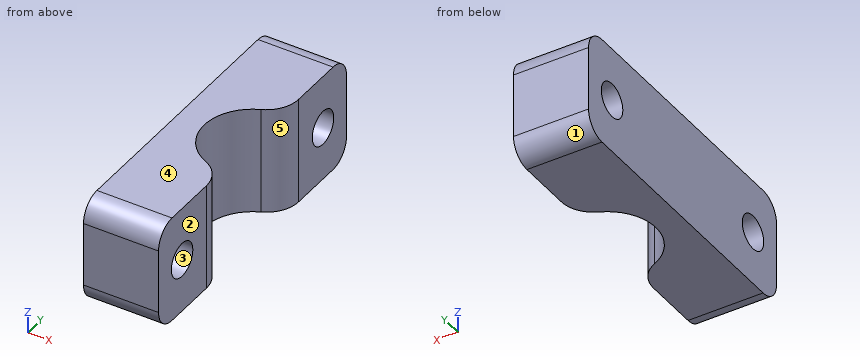
from build123d import *

# Parameters (mm, degrees)
SKETCH1_W               = 12
SKETCH1_H               = 2.1
BOSS_EXTRUDE1_DEPTH     = 3
BOSS_EXTRUDE1_2_DEPTH   = 3
SKETCH2_W               = 4
SKETCH2_H               = 6
BOSS_EXTRUDE2_DEPTH     = 6
SKETCH3_W               = 7
SKETCH3_H               = 28
BOSS_EXTRUDE3_DEPTH     = 5
CUT_EXTRUDE1_DEPTH      = 25.108425983
CUT_EXTRUDE1_DEPTH_BACK = 25.108425983
SKETCH5_R               = 4.5
FILLET1_R               = 3
FILLET2_R               = 2
SKETCH6_R               = 1.6
CUT_EXTRUDE2_DEPTH      = 16
SKETCH7_W               = 18.107499601
SKETCH7_H               = 21.771661969
CUT_EXTRUDE3_DEPTH      = 30


with BuildPart() as part:
    # Sketch1 → Boss-Extrude1 (new, symmetric)
    with BuildSketch(Plane.XY):
        with Locations((0, 1.95)):
            Rectangle(SKETCH1_W, SKETCH1_H)
    extrude(amount=BOSS_EXTRUDE1_DEPTH, both=True)


with BuildPart() as body_2:
    # Sketch1 → Boss-Extrude1 2 (new, symmetric)
    with BuildSketch(Plane.XY):
        with Locations((0, -1.95)):
            Rectangle(SKETCH1_W, SKETCH1_H)
    extrude(amount=BOSS_EXTRUDE1_2_DEPTH, both=True)


with BuildPart() as body_3:
    # Sketch2 → Boss-Extrude2 (new body)
    with BuildSketch(Plane.XY.offset(3)):
        with Locations((8, 0)):
            Rectangle(SKETCH2_W, SKETCH2_H)
    extrude(amount=-BOSS_EXTRUDE2_DEPTH)

    # Sketch3 → Boss-Extrude3 (add, symmetric)
    with BuildSketch(Plane.XY):
        with Locations((13.388345193, 0)):
            Rectangle(SKETCH3_W, SKETCH3_H)
    extrude(amount=BOSS_EXTRUDE3_DEPTH, both=True)

    # Sketch5 → Cut-Extrude1 (cut, two sides: drawn at the far end of the back side and taken through both)
    with BuildSketch(Plane.XY.offset(5).offset(-CUT_EXTRUDE1_DEPTH_BACK)):
        with Locations((16.888345193, 0)):
            Circle(SKETCH5_R)
    extrude(amount=CUT_EXTRUDE1_DEPTH + CUT_EXTRUDE1_DEPTH_BACK, mode=Mode.SUBTRACT)

    # Fillet1
    fillet1_edges = [body_3.edges().sort_by_distance(p)[0] for p in [
        (9.888345193, -3, 0),
        (9.888345193, 3, 0),
        (16.888345193, -4.5, 0),
        (16.888345193, 4.5, 0),
    ]]
    fillet(fillet1_edges, radius=FILLET1_R)

    # Fillet2
    fillet2_edges = [body_3.edges().sort_by_distance(p)[0] for p in [
        (13.388345193, -14, -5),
        (13.388345193, 14, -5),
        (13.388345193, -14, 5),
        (13.388345193, 14, 5),
    ]]
    fillet(fillet2_edges, radius=FILLET2_R)

    # Sketch6 → Cut-Extrude2 (cut)
    with BuildSketch(Plane(origin=(16.888345193, 0, 0), x_dir=(0, 0, -1), z_dir=(1, 0, 0))):
        with Locations((0, 10.5)):
            Circle(SKETCH6_R)
        with Locations((0, -10.5)):
            Circle(SKETCH6_R)
    extrude(amount=-CUT_EXTRUDE2_DEPTH, mode=Mode.SUBTRACT)


with BuildPart() as cut_extrude3_tool:
    # Sketch7 → Cut-Extrude3 (new body)
    with BuildSketch(Plane.XY.offset(5)):
        with Locations((0.834595393, 1.114169015)):
            Rectangle(SKETCH7_W, SKETCH7_H)
    extrude(amount=-CUT_EXTRUDE3_DEPTH)


with BuildPart() as part_1:
    add(part.part)

    # Cut-Extrude3: cut by cut_extrude3_tool
    add(cut_extrude3_tool.part, mode=Mode.SUBTRACT)


with BuildPart() as body_2_1:
    add(body_2.part)

    # Cut-Extrude3: cut by cut_extrude3_tool
    add(cut_extrude3_tool.part, mode=Mode.SUBTRACT)


with BuildPart() as body_3_1:
    add(body_3.part)

    # Cut-Extrude3: cut by cut_extrude3_tool
    add(cut_extrude3_tool.part, mode=Mode.SUBTRACT)


solid = body_3_1.part
Check sheet for the modelled part. Datum: model origin and axes. Units: mm. Face numbers are marked on the shaded views. A direction names the side the tool comes from. Round coordinates to 2 decimals unless told otherwise and drop trailing zeros. Order: outer loops, then holes, each group sorted by start corner. A loop starts at its lowest first (then second) coordinate and runs counter-clockwise, first axis right, second up.
Q1. Cross-section at B-B, the plane x = 16. Enter the section's corners in (y, z), plus the area to 3 significant figures.
Filled sheet:
outline: (-14, -3) arc R2 ccw to (-12, -5) - (-4.74, -5) - (-4.74, 5) - (-12, 5) arc R2 ccw to (-14, 3) - close; (4.74, -5) - (12, -5) arc R2 ccw to (14, -3) - (14, 3) arc R2 ccw to (12, 5) - (4.74, 5) - close; hole circle Ø3.2 at (-10.5, 0); hole circle Ø3.2 at (10.5, 0)
area: 166 mm2
Q2. Cross-section at C-C, the plane z = 0. Enter the section's corners in (x, y).
Filled sheet:
outline: (9.89, -14) - (16.89, -14) - (16.89, -12.1) - (9.89, -12.1) - close; (9.89, -8.9) - (16.89, -8.9) - (16.89, -6.87) arc R3 ccw to (15.09, -4.12) arc R4.5 cw to (15.09, 4.12) arc R3 ccw to (16.89, 6.87) - (16.89, 8.9) - (9.89, 8.9) - close; (9.89, 12.1) - (16.89, 12.1) - (16.89, 14) - (9.89, 14) - close
Q3. Cross-section at A-A, the plane y = -10.5. Enter the section's corners in (x, z), plus the area to 3 significant figures.
Filled sheet:
outline: (9.89, -5) - (16.89, -5) - (16.89, -1.6) - (9.89, -1.6) - close; (9.89, 1.6) - (16.89, 1.6) - (16.89, 5) - (9.89, 5) - close
area: 47.6 mm2
Q4. Cross-section at D-D, the plane x = 11.5. Enter the section's corners in (y, z).
Filled sheet:
outline: (-14, -3) arc R2 ccw to (-12, -5) - (12, -5) arc R2 ccw to (14, -3) - (14, 3) arc R2 ccw to (12, 5) - (-12, 5) arc R2 ccw to (-14, 3) - close; hole circle Ø3.2 at (-10.5, 0); hole circle Ø3.2 at (10.5, 0)
Q5. Set-up check for the marked faces 4 and 5: record each of +Z, -Z, +X, -X, +Y, -Y from which the full face is reachable in a straight line by a thin tool's end or side.
Filled sheet:
face 4: +Z, +X, -X, +Y, -Y
face 5: +Z, -Z, +X
Q6. Scan lines: L1, parallel to Y at x = 11.5, z = 0; L2, parallel to Y at x = 13.75, z = 0; L3, parallel to Y at x = 16, z = -1.25. Record each from-to range of solid material in increasing order.
Filled sheet:
L1: y = -14 to -12.1, -8.9 to 8.9, 12.1 to 14
L2: y = -14 to -12.1, -8.9 to -3.23, 3.23 to 8.9, 12.1 to 14
L3: y = -14 to -11.5, -9.5 to -4.74, 4.74 to 9.5, 11.5 to 14
Q7. Draft check along Z on the marked faces 1, 2 and 3. Enter one of: pulls with the +Z half, pulls with the -Z half, needs draft (parallel to the pull), parting line crosses it, or undercut.
Filled sheet:
face 1: pulls with the -Z half
face 2: needs draft
face 3: undercut
